Answer from the drawing. Dimensions are ordinates in mm from the lowest x, y and z of the part. Coordinates: 2 decimals unless noted, no trailing zeros. Write each loop counter-clockwise with the first axis right and the second up, starting at its lowest first coordinate (ties: lowest second). Pieces come first, ordered by that corner, then holes.
1) The part is cut by section B-B (x = 50). Determine the outline of the cut face in (y, z), then the cut area to 3 significant figures.
2) The part is cut by section C-C (z = 10). Determine the outline of the cut face in (x, y), then the cut area to 3 significant figures.
3) Find the intervals of material crossed by line 1 (Y direction, x = 50, z = 7.5); line 2 (Y direction, x = 22, z = 8.75), in increasing order.
4) Determine the mould class of the marked faces 1 and 2 for opening direction X: +X half, -X half, draft (parallel to the pull), parting line (faces both ways), or undercut.
5) The part is cut by section D-D (x = 73). Determine the outline of the cut face in (y, z).
6) The part is cut by section A-A (y = 150). Determine the outline of the cut face in (x, z), then the cut area to 3 significant figures.
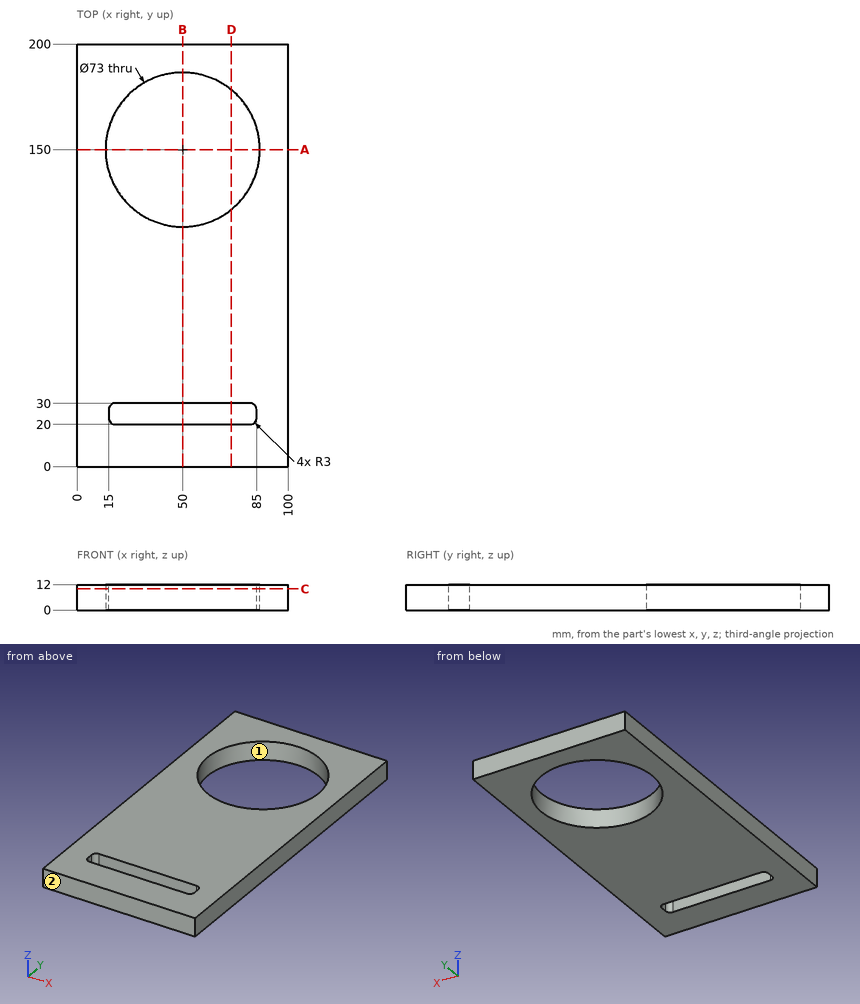
Reported:
1. outline: (0, 0) - (20, 0) - (20, 12) - (0, 12) - close; (30, 0) - (113.5, 0) - (113.5, 12) - (30, 12) - close; (186.5, 0) - (200, 0) - (200, 12) - (186.5, 12) - close
1. area: 1,400 mm2
2. outline: (0, 0) - (100, 0) - (100, 200) - (0, 200) - close; hole circle Ø73 at (50, 150); hole (15, 23) arc R3 ccw to (18, 20) - (82, 20) arc R3 ccw to (85, 23) - (85, 27) arc R3 ccw to (82, 30) - (18, 30) arc R3 ccw to (15, 27) - close
2. area: 15,100 mm2
3. line 1: y = 0 to 20, 30 to 113.5, 186.5 to 200
3. line 2: y = 0 to 20, 30 to 126.59, 173.41 to 200
4. face 1: undercut
4. face 2: draft
5. outline: (0, 0) - (20, 0) - (20, 12) - (0, 12) - close; (30, 0) - (121.66, 0) - (121.66, 12) - (30, 12) - close; (178.34, 0) - (200, 0) - (200, 12) - (178.34, 12) - close
6. outline: (0, 0) - (13.5, 0) - (13.5, 12) - (0, 12) - close; (86.5, 0) - (100, 0) - (100, 12) - (86.5, 12) - close
6. area: 324 mm2
